Could you check a few things on this drawing? It's one solid part, dimensions in mm from its lowest x, y, z. A direction names the side the tool comes from. Give positions to 0.01 mm unless a question says otherwise; leave off trailing zeros. Order: outer loops, then holes, each group sorted by start corner. A loop starts at its lowest first (then second) coordinate and runs counter-clockwise, first axis right, second up. Notation, with made-up numbers: (5.25, -31.75) -> (24.25, -31.75) arc R32 cw to (24.25, -1.75) -> close; hole circle Ø2 at (36.25, 17). An arc over 180 degrees is marked (long way). Answer as a JSON object with one key per item and string values.
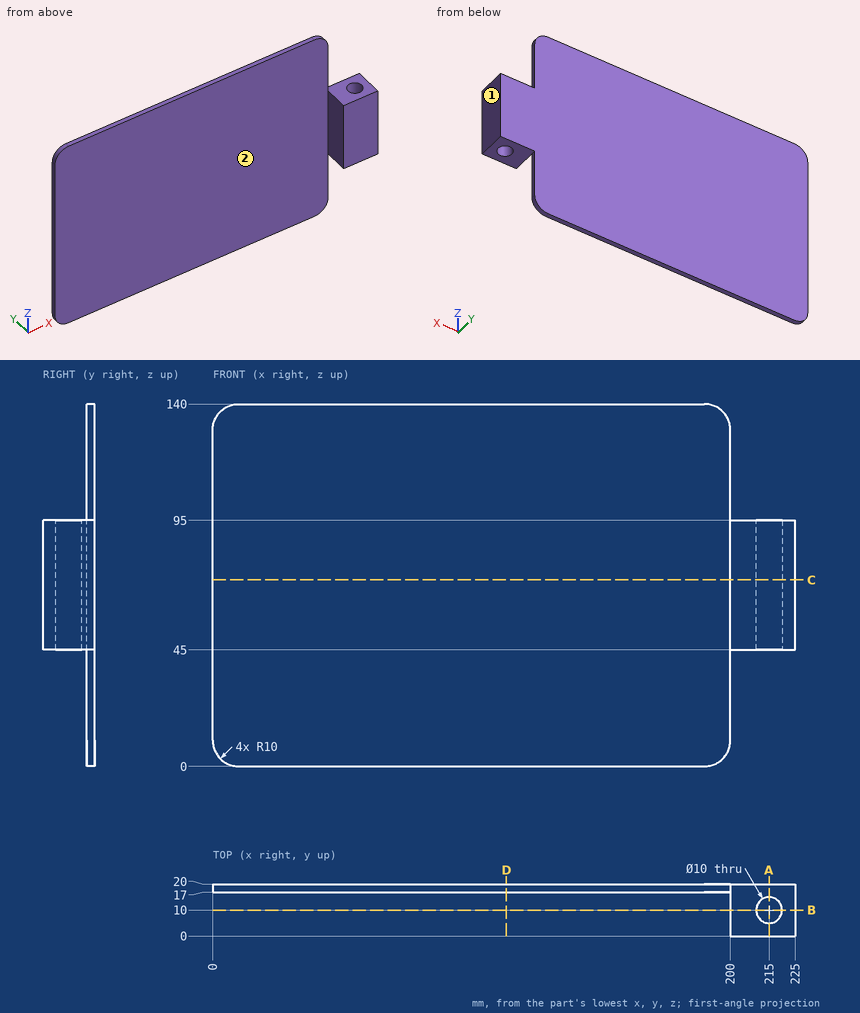
1. Please list where these lines run through material, in increasing order: L1, parallel to Y at x = 215, z = 76; L2, parallel to Y at x = 114.5, z = 74; L3, parallel to Y at x = 213, z = 72.
Worked answers:
{"L1": "0 to 5, 15 to 20", "L2": "17 to 20", "L3": "0 to 5.42, 14.58 to 20"}
2. If we section it at A-A on x = 215: Please give me the cut outline in (y, z), then the cut area to 3 significant figures.
Worked answers:
{"outline": "(0, 45) -> (5, 45) -> (5, 95) -> (0, 95) -> close; (15, 45) -> (20, 45) -> (20, 95) -> (15, 95) -> close", "area": "500 mm²"}
3. Will these pins go through, and if not, where does the flat tip stop? pin 1 Ø12 at (x, z) = (41.5, 109.5) entering from -Y; pin 2 Ø2.5 at (y, z) = (19, 27.5) entering from +X; pin 3 Ø8 at (x, y) = (91.5, 17.5) entering from -Z.
Worked answers:
{"pin 1": "y = 17", "pin 2": "x = 200", "pin 3": "z = 0"}
4. If we section it at C-C on z = 72: Please give me the cut outline in (x, y), then the cut area to 3 significant figures.
Worked answers:
{"outline": "(0, 17) -> (200, 17) -> (200, 0) -> (225, 0) -> (225, 20) -> (0, 20) -> close; hole circle Ø10 at (215, 10)", "area": "1,020 mm²"}
5. If we section it at B-B on y = 10: Please give me the cut outline in (x, z).
Worked answers:
{"outline": "(200, 45) -> (210, 45) -> (210, 95) -> (200, 95) -> close; (220, 45) -> (225, 45) -> (225, 95) -> (220, 95) -> close"}
6. If we section it at D-D on x = 113.5: Please give me the cut outline in (y, z).
Worked answers:
{"outline": "(17, 0) -> (20, 0) -> (20, 140) -> (17, 140) -> close"}
7. For the marked faces 1 and 2, which set-ups out of +Z, -Z, +X, -X, +Y, -Y let a thin tool reach every point of the face, with its end or its side?
Worked answers:
{"face 1": "+Z, -Z, +X, +Y, -Y", "face 2": "+Z, -Z, -X, -Y"}
